```python
from build123d import *

# Parameters (mm, degrees)
ESQUISSE1_W             = 65
ESQUISSE1_H             = 125
BOSS_EXTRU_1_DEPTH      = 80
COQUE1_T                = -3
ESQUISSE2_OUTSIDE_W     = 159.404
ESQUISSE2_OUTSIDE_H     = 114.404
ENL_V_MAT_EXTRU_1_DEPTH = 66
CONG_2_R                = 5
CONG_3_R                = 2
CHANFREIN1_SIZE         = 1
ESQUISSE3_R             = 15.24
ENL_V_MAT_EXTRU_2_DEPTH = 0.1


with BuildPart() as part:
    # Esquisse1 → Boss.-Extru.1 (new body)
    with BuildSketch(Plane(origin=(0, 0, 0), x_dir=(1, 0, 0), z_dir=(0, 1, 0))):
        Rectangle(ESQUISSE1_W, ESQUISSE1_H)
    extrude(amount=BOSS_EXTRU_1_DEPTH)

    # Coque1
    coque1_openings = [part.faces().sort_by_distance(p)[0] for p in [
        (0, 0, 0),
    ]]
    offset(amount=COQUE1_T, openings=coque1_openings, kind=Kind.INTERSECTION)

    # Esquisse2 outside → Enlèv. mat.-Extru.1 (cut, through all)
    with BuildSketch(Plane(origin=(32.5, 0, 0), x_dir=(0, 0, -1), z_dir=(1, 0, 0))):
        with Locations((0, 40)):
            Rectangle(ESQUISSE2_OUTSIDE_W, ESQUISSE2_OUTSIDE_H)
        Polygon((-47.5, 80), (-47.5, 72), (27.5, 15), (62.5, 15), (62.5, 80), align=None, mode=Mode.SUBTRACT)
    extrude(amount=-ENL_V_MAT_EXTRU_1_DEPTH, mode=Mode.SUBTRACT)

    # Congé2
    cong_2_edges = [part.edges().sort_by_distance(p)[0] for p in [
        (-32.5, 47.5, -62.5),
        (32.5, 47.5, -62.5),
    ]]
    fillet(cong_2_edges, radius=CONG_2_R)

    # Congé3
    cong_3_edges = [part.edges().sort_by_distance(p)[0] for p in [
        (29.5, 46, -59.5),
        (-29.5, 46, -59.5),
    ]]
    fillet(cong_3_edges, radius=CONG_3_R)

    # Chanfrein1
    chanfrein1_edges = [part.edges().sort_by_distance(p)[0] for p in [
        (32.5, 80, -5),
        (-32.5, 80, -5),
        (0, 80, -62.5),
        (31.035533906, 80, -61.035533906),
        (-31.035533906, 80, -61.035533906),
    ]]
    chamfer(chanfrein1_edges, length=CHANFREIN1_SIZE)

    # Esquisse3 → Enlèv. mat.-Extru.2 (cut)
    with BuildSketch(Plane(origin=(0, 0, -62.5), x_dir=(-1, 0, 0), z_dir=(0, 0, -1))):
        with Locations((0, 55)):
            Circle(ESQUISSE3_R)
    extrude(amount=-ENL_V_MAT_EXTRU_2_DEPTH, mode=Mode.SUBTRACT)


solid = part.part
```
Source: CAD feature listing. Evaluate the final solid. Frame: model axes, mm. A direction names the side the tool comes from. Round coordinates to 2 decimals unless told otherwise and drop trailing zeros. Loops run counter-clockwise (first coordinate to the right, second up) from the corner with the lowest first, then second, coordinate; pieces in that order, holes last.
1. Contact query for flat-ended pins moving along their axis: pin 1 (2 mm diameter, centred on x = -10, z = -18, fed in from -Y); pin 2 (16.5 mm diameter, centred on x = 2.5, y = 50, fed in from +Z); pin 3 (24.5 mm diameter, centred on x = 0, y = 55, fed in from -Z). Output: stop coordinate, or through.
2. Section query B-B on y = 74.5. Output: boundary loops of the cut face in (x, z), and give its area (3 significant figures).
3. Ray query, L1, parallel to X at y = 51, z = -36; L2, parallel to Z at x = 16, y = 38; L3, parallel to Y at x = 9.5, z = -1.5. Return the intervals inside material, ascending.
4. Section query C-C on x = 0. Output: boundary loops of the cut face in (y, z), and give its area (3 significant figures).
5. Mould query, pull axis X, two halves, no side actions, for faces 4 (the cylindrical face through (31, 47.45, -61.07)), 5 (the flat face through (0, 77, -7)), 6 (the flat face through (-32.5, 54, -16)), 7 (the flat face through (0.2, 79.6, 47.5)). Classes: released by +X, released by -X, zero draft, split by the parting line, or undercut.
6. Section query D-D on z = 20. Output: boundary loops of the cut face in (x, y).
7. Section query A-A on z = -22. Output: boundary loops of the cut face in (x, y), and give its area (3 significant figures).
8. Access query for faces 1 (the flat face through (-29.5, 52, -16)), 2 (the flat face through (0, 55, -62.4)), 3 (the cylindrical face through (-31.07, 47.45, -61)). Directions: +Z, -Z, +X, -X, +Y, -Y. A direction counts if a zero-diameter tool reaches every point of the face in a straight line with its end or side. Return the directions, or none.
Answers below:
1. pin 1: stops at y = 77
1. pin 2: stops at z = -59.5
1. pin 3: stops at z = -62.4
2. outline: (-32.5, -57.5) arc R5 ccw to (-27.5, -62.5) - (27.5, -62.5) arc R5 ccw to (32.5, -57.5) - (32.5, 47.5) - (29.5, 47.5) - (29.5, -57.5) arc R2 cw to (27.5, -59.5) - (-27.5, -59.5) arc R2 cw to (-29.5, -57.5) - (-29.5, 47.5) - (-32.5, 47.5) - close
2. area: 828 mm2
3. L1: x = -32.5 to -29.5, 29.5 to 32.5
3. L2: z = -62.5 to -59.5
3. L3: y = 77 to 80
4. outline: (15, -62.5) - (39.76, -62.5) - (39.76, -62.4) - (70.24, -62.4) - (70.24, -62.5) - (79, -62.5) - (80, -61.5) - (80, 47.5) - (77, 47.5) - (77, -59.5) - (15, -59.5) - close
4. area: 512 mm2
5. face 4: released by +X
5. face 5: undercut
5. face 6: released by -X
5. face 7: zero draft
6. outline: (-32.5, 51.1) - (-29.5, 51.1) - (-29.5, 77) - (29.5, 77) - (29.5, 51.1) - (32.5, 51.1) - (32.5, 79) - (31.5, 80) - (-31.5, 80) - (-32.5, 79) - close
7. outline: (-32.5, 19.18) - (-29.5, 19.18) - (-29.5, 77) - (29.5, 77) - (29.5, 19.18) - (32.5, 19.18) - (32.5, 79) - (31.5, 80) - (-31.5, 80) - (-32.5, 79) - close
7. area: 541 mm2
8. face 1: +Z, -Y
8. face 2: -Z
8. face 3: -Z, -X, +Y, -Y
